Verification items for this drawing (mm, ordinates from the low corner). A direction names the side the tool comes from. Round coordinates to 2 decimals unless told otherwise and drop trailing zeros. Loops run counter-clockwise (first coordinate to the right, second up) from the corner with the lowest first, then second, coordinate; pieces in that order, holes last. Notation, with made-up numbers: (82, -34) - (111, -34) arc R21 ccw to (111, -7) - close; hole circle Ø2 at (70.5, 12). An arc over 180 degrees is marked (long way). Answer in a Markdown table with one row per item. Add a question column.
(1) Thickness scan on line 1 along X through (y, z) = (2.25, 3.81); line 2 along Y through (x, z) = (8, 3) (1 decimal); line 3 along X through (y, z) = (1.5, 5.25). Record the ranges inside material, lowest first.
(2) Cross-section at B-B on x = 5. Enter the section's corners in (y, z) (1 decimal).
(3) Gauge pin test, flat ends, axial feed: pin 1 (4 mm diameter, centred on x = 6, z = 5, fed in from -Y); pin 2 (0.5 mm diameter, centred on y = 0.5, z = 3.5, fed in from -X). Record the tip position at first contact, or that the pin passes through.
(4) Mould release check, pull along Y, two halves, no side actions. Record for the marked faces 4, 5 and 6: +Y half, -Y half, draft (parallel to the pull), parting line (faces both ways), or undercut.
(5) Cross-section at D-D on y = 5.5. Enter the section's corners in (x, z).
(6) Access from +Z, -Z, +X, -X, +Y, -Y to the whole of each face (thin tool, end or side, straight path). Record for the marked faces 1, 2 and 3.
(7) Cross-section at C-C on y = 1.5. Enter the section's corners in (x, z), then the cut area to 3 significant figures.
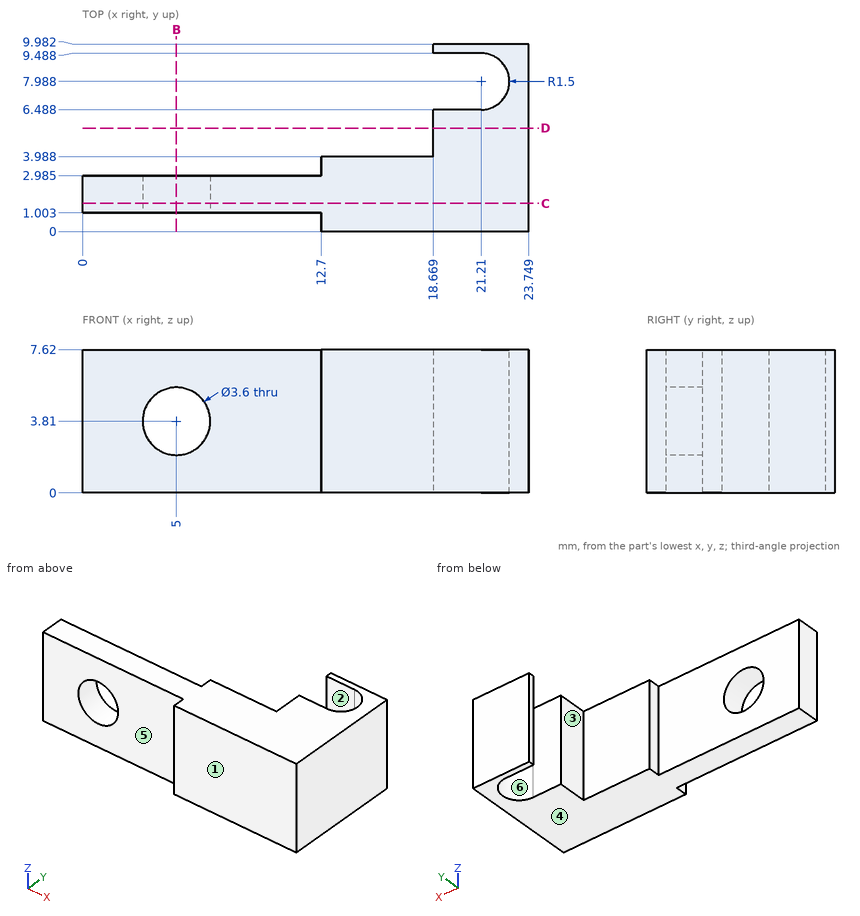
Answers:
| question | item | result |
|---|---|---|
| 1 | line 1 | x = 0 to 3.2, 6.8 to 23.75 |
| 1 | line 2 | y = 1 to 3 |
| 1 | line 3 | x = 0 to 3.92, 6.08 to 23.75 |
| 2 | outline | (1, 0) - (3, 0) - (3, 2) - (1, 2) - close; (1, 5.6) - (3, 5.6) - (3, 7.6) - (1, 7.6) - close |
| 3 | pin 1 | stops at y = 1 |
| 3 | pin 2 | stops at x = 12.7 |
| 4 | face 4 | draft |
| 4 | face 5 | -Y half |
| 4 | face 6 | undercut |
| 5 | outline | (18.67, 0) - (23.75, 0) - (23.75, 7.62) - (18.67, 7.62) - close |
| 6 | face 1 | +Z, -Z, +X, -X, -Y |
| 6 | face 2 | +Z, -Z, -X |
| 6 | face 3 | +Z, -Z, -X, +Y |
| 7 | outline | (0, 0) - (23.75, 0) - (23.75, 7.62) - (0, 7.62) - close; hole circle Ø3.6 at (5, 3.81) |
| 7 | area | 171 mm^2 |
